CAD build for the part. Positions are in the model's coordinates, mm. A direction names the side the tool comes from. Give positions to 0.01 mm unless a question says otherwise; leave off trailing zeros. Order: outer loops, then holes, each group sorted by start corner. A loop starts at its lowest first (then second) coordinate and runs counter-clockwise, first axis right, second up.
from build123d import *

# Parameters (mm, degrees)
PAD_DEPTH        = 4
HOLE_D           = 3
HOLE_DEPTH       = 25
HOLE_CSINK_D     = 6.1
HOLE_CSINK_ANGLE = 90
SKETCH002_R      = 4
PAD001_DEPTH     = 6
SKETCH003_W      = 40
SKETCH003_H      = 5
PAD002_DEPTH     = 1
SKETCH004_W      = 30
SKETCH004_H      = 64
SKETCH004_H_2    = 60
SKETCH004_W_2    = 44
SKETCH004_H_3    = 8
POCKET_DEPTH     = 2


with BuildPart() as part:
    # Sketch → Pad (new body)
    with BuildSketch(Plane.XY):
        with BuildLine():
            Line((60, -32), (60, 32))
            ThreePointArc((60, 32), (58.242641, 36.242641), (54, 38))
            Line((54, 38), (-54, 38))
            ThreePointArc((-54, 38), (-58.242641, 36.242641), (-60, 32))
            Line((-60, 32), (-60, -32))
            ThreePointArc((-60, -32), (-58.242641, -36.242641), (-54, -38))
            Line((-54, -38), (54, -38))
            ThreePointArc((54, -38), (58.242641, -36.242641), (60, -32))
        make_face()
    extrude(amount=PAD_DEPTH)

    # Hole
    with Locations(Plane.XY.offset(4)):
        with Locations((0, -35), (0, 35), (50, 35), (-50, 35), (-50, -35), (50, -35)):
            CounterSinkHole(HOLE_D / 2, HOLE_CSINK_D / 2, depth=HOLE_DEPTH, counter_sink_angle=HOLE_CSINK_ANGLE)

    # Sketch002 (on Face4 of Hole) → Pad001 (join)
    with BuildSketch(Plane(origin=(0, 0, 0), x_dir=(1, 0, 0), z_dir=(0, 0, -1))):
        with Locations((18, 0)):
            Circle(SKETCH002_R)
        with Locations((-18, 0)):
            Circle(SKETCH002_R)
    extrude(amount=PAD001_DEPTH)

    # Sketch003 (on Face4 of Pad001) → Pad002 (join)
    with BuildSketch(Plane(origin=(0, 0, 0), x_dir=(1, 0, 0), z_dir=(0, 0, -1))):
        with Locations((0, 21.5)):
            Rectangle(SKETCH003_W, SKETCH003_H)
        with Locations((0, -21.5)):
            Rectangle(SKETCH003_W, SKETCH003_H)
    extrude(amount=PAD002_DEPTH)

    # Sketch004 (on Face4 of Pad002) → Pocket (cut)
    with BuildSketch(Plane(origin=(0, 0, 0), x_dir=(1, 0, 0), z_dir=(0, 0, -1))):
        with Locations((-42, 0)):
            Rectangle(SKETCH004_W, SKETCH004_H)
        with Locations((42, 2)):
            Rectangle(SKETCH004_W, SKETCH004_H_2)
        with Locations((0, 11)):
            Rectangle(SKETCH004_W_2, SKETCH004_H_3)
        with Locations((0, -11)):
            Rectangle(SKETCH004_W_2, SKETCH004_H_3)
    extrude(amount=-POCKET_DEPTH, mode=Mode.SUBTRACT)


solid = part.part
1. 3-axis set-ups, long thin cutter, end or side, ignore diameter. For faces 4 (the cylindrical face through (58.289, 36.196, 1.972)), 5 (the flat face through (0, 21, -1)), 6 (the cylindrical face through (-21.2, 2.4, -3)): which of +Z, -Z, +X, -X, +Y, -Y reach the whole face in a straight line?
2. Saw through at D-D on x = 18. Give the cut face in (y, z).
3. Saw through at C-C on z = -2.75. Give the cut face in (x, y), plus the area to 3 significant figures.
4. Mould opens along Y. For faces 1 (the flat face through (-18, 0, -6)), 2 (the cylindrical face through (-58.289, -36.196, 1.972)), 3 (the cylindrical face through (51.2, -35.9, 1.2)) say: released by +Y, released by -Y, zero draft, split by the parting line, or undercut.
5. Pin check, flat tips, straight feed: P1, Ø2.5, axis at x = 7.5, y = -20.5, coming from the -Z side; P2, Ø0.5, axis at y = -21.5, z = -0.5, coming from the +X side; P3, Ø1.5, axis at x = 24.5, y = 24.5, coming from the -Z side. Stop position of each tip, or through.
6. Saw through at B-B on y = 0. Give the cut face in (x, z).
7. Saw through at A-A on x = 34. Give the cut face in (y, z), plus the area to 3 significant figures.
8. Wall check: line 1 (X direction, y = -25.5, z = 1.75); line 2 (Y direction, x = -50, z = 0.9); line 3 (X direction, y = -35, z = 1.2). Give the ranges that are in metal, low to high.
Reported:
1. face 4: +Z, -Z, +X, +Y
1. face 5: -Z, +X, -X, +Y
1. face 6: -Z
2. outline: (-38, 0) - (-24, 0) - (-24, -1) - (-19, -1) - (-19, 0) - (-15, 0) - (-15, 2) - (-7, 2) - (-7, 0) - (-4, 0) - (-4, -6) - (4, -6) - (4, 0) - (7, 0) - (7, 2) - (15, 2) - (15, 0) - (19, 0) - (19, -1) - (24, -1) - (24, 0) - (38, 0) - (38, 4) - (-38, 4) - close
3. outline: circle Ø8 at (-18, 0); circle Ø8 at (18, 0)
3. area: 101 mm2
4. face 1: zero draft
4. face 2: released by -Y
4. face 3: undercut
5. P1: stops at z = -1
5. P2: stops at x = 20
5. P3: stops at z = 0
6. outline: (-60, 0) - (-57, 0) - (-57, 2) - (-27, 2) - (-27, 0) - (-22, 0) - (-22, -6) - (-14, -6) - (-14, 0) - (14, 0) - (14, -6) - (22, -6) - (22, 0) - (27, 0) - (27, 2) - (57, 2) - (57, 0) - (60, 0) - (60, 4) - (-60, 4) - close
7. outline: (-38, 0) - (-32, 0) - (-32, 2) - (28, 2) - (28, 0) - (38, 0) - (38, 4) - (-38, 4) - close
7. area: 184 mm2
8. line 1: x = -60 to -57, -27 to 27, 57 to 60
8. line 2: y = -38 to -36.5, -33.5 to -32, 32 to 33.5, 36.5 to 38
8. line 3: x = -59.2 to -51.5, -48.5 to -1.5, 1.5 to 48.5, 51.5 to 59.2
